Autodesk Inventor part; units mm, degrees
ref_plane "YZ Plane" through (0, 0, 0) normal (1, 0, 0) x (0, 1, 0)
ref_plane "XZ Plane" through (0, 0, 0) normal (0, 1, 0) x (-1, 0, 0)
ref_plane "XY Plane" through (0, 0, 0) normal (0, 0, 1) x (1, 0, 0)
sketch "Sketch1" plane through (0, 0, 0) normal (0, 1, 0) x (-1, 0, 0)
  circle A0 centre (0, 0) radius 203.2
  dimension "d0" = 406.4
extrude "Extrusion1" add sketch "Sketch1" along normal blind 4.7625
sketch "Sketch6" plane through (0, 0, 0) normal (0, -1, 0) x (1, 0, 0)
  point P0 (0, 0)
  point P1 (52.197, 152.4)
  point P2 (-52.197, 152.4)
  dimension "d48" = 0
  dimension "d49" = 104.394
  dimension "d50" = 52.197
  dimension "d51" = 152.4
hole "Hole3" at (52.197, 0, 152.4) at (-52.197, 0, 152.4) direction (0, 1, 0) diameter 4.4958 end through all
sketch "Sketch8" plane through (0, 4.7625, 0) normal (0, 1, 0) x (1, 0, 0)
  line L0 (-249.9736, 258.2829) -> (238.9858, 258.2829)
  line L1 (238.9858, 258.2829) -> (238.9858, 152.4)
  line L2 (238.9858, 152.4) -> (-249.9736, 152.4)
  line L3 (-249.9736, 152.4) -> (-249.9736, 258.2829)
  point P0 (0, 0)
  dimension "d80" = 152.4
extrude "Extrusion4" cut sketch "Sketch8" against normal blind 100.0125
sketch "Sketch14" plane through (0, 4.7625, 0) normal (0, 1, 0) x (1, 0, 0)
  circle A0 centre (52.197, -152.4) radius 2.2479
  circle A1 centre (-52.197, -152.4) radius 2.2479
  point P0 (0, 0)
  point P1 (-52.197, 29.87)
  point P2 (52.197, 29.87)
  dimension "d138" = 0
  dimension "d139" = 182.27
  dimension "d140" = 182.27
  dimension "d141" = 0
hole "Hole7" at (-52.197, 4.7625, -29.87) at (52.197, 4.7625, -29.87) direction (0, -1, 0) diameter 4.4958 depth 25.4 tip angle 118
sketch "Sketch15" plane through (0, 4.7625, 0) normal (0, 1, 0) x (1, 0, 0)
  circle A0 centre (-52.197, -152.4) radius 2.2479
  point P0 (0, 0)
  point P1 (-78.74, -165.1)
  point P2 (-78.74, -38.1)
  point P3 (78.74, -165.1)
  point P4 (78.74, -38.1)
  dimension "d149" = 0
  dimension "d150" = 0
  dimension "d151" = 0
  dimension "d152" = 0
  dimension "d153" = 127
  dimension "d155" = 157.48
  dimension "d156" = 78.74
  dimension "d270" = 12.7
hole "Hole8" at (-78.74, 4.7625, 165.1) at (-78.74, 4.7625, 38.1) at (78.74, 4.7625, 165.1) at (78.74, 4.7625, 38.1) direction (0, -1, 0) diameter 4.4958 end through all
sketch "Sketch16" plane through (0, 4.7625, 0) normal (0, 1, 0) x (1, 0, 0)
  circle A0 centre (78.74, -165.1) radius 2.2479
  point P0 (0, 0)
  point P1 (81.28, -96.647)
  point P2 (129.032, -96.647)
  point P3 (81.28, -139.7)
  point P4 (129.032, -139.7)
  dimension "d164" = 0
  dimension "d165" = 0
  dimension "d166" = 0
  dimension "d167" = 0
  dimension "d170" = 47.752
  dimension "d171" = 43.053
  dimension "d271" = 2.54
  dimension "d272" = 25.4
hole "Hole9" at (81.28, 4.7625, 96.647) at (129.032, 4.7625, 96.647) at (81.28, 4.7625, 139.7) at (129.032, 4.7625, 139.7) direction (0, -1, 0) diameter 4.4958 end through all
sketch "Sketch17" plane through (0, 4.7625, 0) normal (0, 1, 0) x (1, 0, 0)
  circle A0 centre (-52.197, 29.87) radius 2.2479
  point P0 (0, 0)
  point P1 (-29.5275, 102.9204)
  point P2 (-29.5275, 42.57)
  point P3 (29.5275, 42.57)
  point P4 (29.5275, 102.9204)
  dimension "d179" = 0
  dimension "d180" = 0
  dimension "d181" = 0
  dimension "d182" = 0
  dimension "d183" = 59.055
  dimension "d184" = 29.5275
  dimension "d185" = 12.7
  dimension "d186" = 60.3504
hole "Hole10" at (-29.5275, 4.7625, -102.9204) at (-29.5275, 4.7625, -42.57) at (29.5275, 4.7625, -42.57) at (29.5275, 4.7625, -102.9204) direction (0, -1, 0) diameter 4.4958 end through all
sketch "Sketch18" plane through (0, 4.7625, 0) normal (0, 1, 0) x (1, 0, 0)
  line L0 (134.4042, 152.4) -> (-134.4042, 152.4)
  point P0 (0, 0)
  point P1 (-45.085, 144.78)
  point P2 (45.085, 144.78)
  point P3 (45.085, 125.73)
  point P4 (-45.085, 125.73)
  dimension "d194" = 90.17
  dimension "d195" = 0
  dimension "d196" = 19.05
  dimension "d197" = 0
  dimension "d198" = 0
  dimension "d199" = 0
  dimension "d200" = 7.62
  dimension "d201" = 45.085
hole "Hole11" at (-45.085, 4.7625, -144.78) at (45.085, 4.7625, -144.78) at (45.085, 4.7625, -125.73) at (-45.085, 4.7625, -125.73) direction (0, -1, 0) diameter 4.4958 end through all
sketch "Sketch19" plane through (0, 4.7625, 0) normal (0, 1, 0) x (1, 0, 0)
  point P0 (0, 0)
  point P1 (-106.68, -76.2)
  point P2 (-121.92, -76.2)
  point P3 (106.68, -76.2)
  point P4 (121.92, -76.2)
  dimension "d209" = 0
  dimension "d210" = 76.2
  dimension "d211" = 76.2
  dimension "d212" = 0
  dimension "d213" = 15.24
  dimension "d214" = 15.24
  dimension "d215" = 106.68
  dimension "d216" = 106.68
hole "Hole12" at (-106.68, 4.7625, 76.2) at (-121.92, 4.7625, 76.2) at (106.68, 4.7625, 76.2) at (121.92, 4.7625, 76.2) direction (0, -1, 0) diameter 5.1054 depth 25.4 tip angle 118
sketch "Sketch20" plane through (0, 4.7625, 0) normal (0, 1, 0) x (1, 0, 0)
  circle A0 centre (-121.92, -76.2) radius 2.5527
  circle A1 centre (-106.68, -76.2) radius 2.5527
  circle A2 centre (106.68, -76.2) radius 2.5527
  circle A3 centre (121.92, -76.2) radius 2.5527
  circle A4 centre (121.92, -76.2) radius 2.5527
  point P0 (0, 0)
  point P1 (-121.92, 25.4)
  point P2 (-106.68, 25.4)
  point P3 (121.92, 25.4)
  point P4 (106.68, 25.4)
  dimension "d224" = 0
  dimension "d225" = 0
  dimension "d226" = 0
  dimension "d227" = 0
  dimension "d228" = 0
  dimension "d229" = 0
  dimension "d230" = 0
  dimension "d231" = 101.6
hole "Hole13" at (-121.92, 4.7625, -25.4) at (-106.68, 4.7625, -25.4) at (121.92, 4.7625, -25.4) at (106.68, 4.7625, -25.4) direction (0, -1, 0) diameter 4.4958 end through all
sketch "Sketch21" plane through (0, 4.7625, 0) normal (0, 1, 0) x (1, 0, 0)
  circle A0 centre (121.92, 25.4) radius 2.2479
  circle A1 centre (106.68, 25.4) radius 2.2479
  circle A2 centre (-106.68, 25.4) radius 2.2479
  circle A3 centre (-121.92, 25.4) radius 2.2479
  point P0 (0, 0)
  point P1 (-87.63, 25.4)
  point P2 (-185.42, 25.4)
  point P3 (87.63, 25.4)
  point P4 (185.42, 25.4)
  dimension "d239" = 0
  dimension "d240" = 0
  dimension "d241" = 0
  dimension "d242" = 0
  dimension "d243" = 19.05
  dimension "d244" = 63.5
  dimension "d245" = 63.5
  dimension "d246" = 19.05
hole "Hole14" at (-87.63, 4.7625, -25.4) at (-185.42, 4.7625, -25.4) at (87.63, 4.7625, -25.4) at (185.42, 4.7625, -25.4) direction (0, -1, 0) diameter 4.4958 end through all
sketch "Sketch22" plane through (0, 4.7625, 0) normal (0, 1, 0) x (1, 0, 0)
  circle A0 centre (-121.92, -76.2) radius 2.5527
  circle A1 centre (-106.68, -76.2) radius 2.5527
  circle A2 centre (106.68, -76.2) radius 2.5527
  circle A3 centre (121.92, -76.2) radius 2.5527
  point P0 (0, 0)
  point P1 (-140.97, -76.2)
  point P2 (-166.37, -76.2)
  point P3 (140.97, -76.2)
  point P4 (166.37, -76.2)
  dimension "d254" = 0
  dimension "d255" = 0
  dimension "d256" = 19.05
  dimension "d257" = 25.4
  dimension "d258" = 0
  dimension "d259" = 0
  dimension "d260" = 25.4
  dimension "d261" = 19.05
hole "Hole15" at (-140.97, 4.7625, 76.2) at (-166.37, 4.7625, 76.2) at (140.97, 4.7625, 76.2) at (166.37, 4.7625, 76.2) direction (0, -1, 0) diameter 4.4958 end through all
sketch "Sketch23" plane through (0, 4.7625, 0) normal (0, 1, 0) x (1, 0, 0)
  line L0 (75.8881, -46.5788) -> (84.511, -46.5788)
  line L1 (87.686, -49.7538) -> (87.686, -83.9555)
  line L2 (84.511, -87.1305) -> (75.8881, -87.1305)
  line L3 (72.7131, -83.9555) -> (72.7131, -49.7538)
  arc A0 (87.686, -49.7538) -> (84.511, -46.5788) centre (84.511, -49.7538) ccw
  arc A1 (84.511, -87.1305) -> (87.686, -83.9555) centre (84.511, -83.9555) ccw
  arc A2 (72.7131, -83.9555) -> (75.8881, -87.1305) centre (75.8881, -83.9555) ccw
  arc A3 (75.8881, -46.5788) -> (72.7131, -49.7538) centre (75.8881, -49.7538) ccw
  point P0 (0, 0)
  dimension "d273" = 3.175
extrude "Extrusion8" cut sketch "Sketch23" against normal blind 25.4
sketch "Sketch24" plane through (0, 4.7625, 0) normal (0, 1, 0) x (1, 0, 0)
  circle A0 centre (-78.74, -165.1) radius 2.2479
  point P0 (0, 0)
  point P1 (-133.35, -99.06)
  point P2 (-72.39, -99.06)
  point P3 (-133.35, -139.7)
  point P4 (-72.39, -139.7)
  dimension "d276" = 40.64
  dimension "d277" = 60.96
  dimension "d278" = 0
  dimension "d279" = 0
  dimension "d280" = 0
  dimension "d281" = 0
  dimension "d289" = 25.4
  dimension "d290" = 6.35
hole "Hole16" at (-133.35, 4.7625, 99.06) at (-72.39, 4.7625, 99.06) at (-72.39, 4.7625, 139.7) at (-133.35, 4.7625, 139.7) direction (0, -1, 0) diameter 4.4958 end through all
sketch "Sketch25" plane through (0, 0, 0) normal (0, -1, 0) x (1, 0, 0)
  point P0 (0, 0)
  point P1 (-101.6, -50.8)
  point P2 (-101.6, -127)
  point P3 (101.6, -127)
  point P4 (101.6, -50.8)
  dimension "d291" = 0
  dimension "d292" = 0
  dimension "d293" = 0
  dimension "d294" = 0
  dimension "d295" = 101.6
  dimension "d296" = 101.6
  dimension "d297" = 76.2
  dimension "d298" = 50.8
hole "Hole17" at (-101.6, 0, -50.8) at (-101.6, 0, -127) at (101.6, 0, -127) at (101.6, 0, -50.8) direction (0, 1, 0) diameter 4.4958 end through all
sketch "Sketch26" plane through (0, 4.7625, 0) normal (0, 1, 0) x (1, 0, 0)
  circle A0 centre (-166.37, -76.2) radius 2.2479
  circle A1 centre (166.37, -76.2) radius 2.2479
  point P0 (0, 0)
  point P1 (-166.37, -91.44)
  point P2 (-147.32, -91.44)
  point P3 (166.37, -95.25)
  point P4 (147.32, -95.25)
  dimension "d306" = 0
  dimension "d307" = 15.24
  dimension "d308" = 0
  dimension "d309" = 19.05
  dimension "d310" = 0
  dimension "d311" = 19.05
  dimension "d312" = 0
  dimension "d313" = 19.05
hole "Hole18" at (-166.37, 4.7625, 91.44) at (-147.32, 4.7625, 91.44) at (147.32, 4.7625, 95.25) at (166.37, 4.7625, 95.25) direction (0, -1, 0) diameter 4.4958 end through all
properties part number "TopPlate"
Geometry: final body of the model. Coordinates: model frame, mm. Round coordinates to 2 decimals unless told otherwise and drop trailing zeros. Order: outer loops, then holes, each group sorted by start corner. A loop starts at its lowest first (then second) coordinate and runs counter-clockwise, first axis right, second up. Notation, with made-up numbers: (78, 85.25) - (108, 85.25) arc R13 cw to (108, 107.25) - close; hole circle Ø3 at (-24.5, 28). An arc over 180 degrees is marked (long way). Write item = value, one per line. Start each with the question number.
Q1. Cut plane A-A on z = -71. Return the cut outline in (x, y).
Q2. Pin query (flat end, axial travel): pin 1 (2.5 mm diameter, centred on y = 1.5, z = 73.5, fed in from +X); pin 2 (2 mm diameter, centred on y = 3, z = -20, fed in from -X). Return the tip coordinate at first contact, or that it passes through.
Q3. Cut plane B-B on y = 3.45. Give the number of separate pieces and of enclosed holes in the cut face, and give its area (3 significant figures).
Q4. Ray query, line 1 (X direction, y = 1.8, z = 95.25); line 2 (Z direction, x = 78.74, y = 1.45); line 3 (Z direction, x = 81.28, y = 1.8). Return the intervals inside material, ascending. Write a range as from..to.
Outcome:
q1.outline = (-190.39, 0) - (190.39, 0) - (190.39, 4.76) - (-190.39, 4.76) - close
q2.pin_1 = 189.92
q2.pin_2 = -202.31
q3.separate_pieces = 1
q3.enclosed_holes = 49
q3.area = 119,000 mm^2
q4.line_1 = -179.49..79.52, 83.04..127.27, 130.79..145.07, 149.57..164.12, 168.62..179.49
q4.line_2 = -152.4..35.85, 40.35..46.58, 87.13..162.85, 167.35..187.32
q4.line_3 = -152.4..46.58, 87.13..94.4, 98.89..137.45, 141.95..186.24
